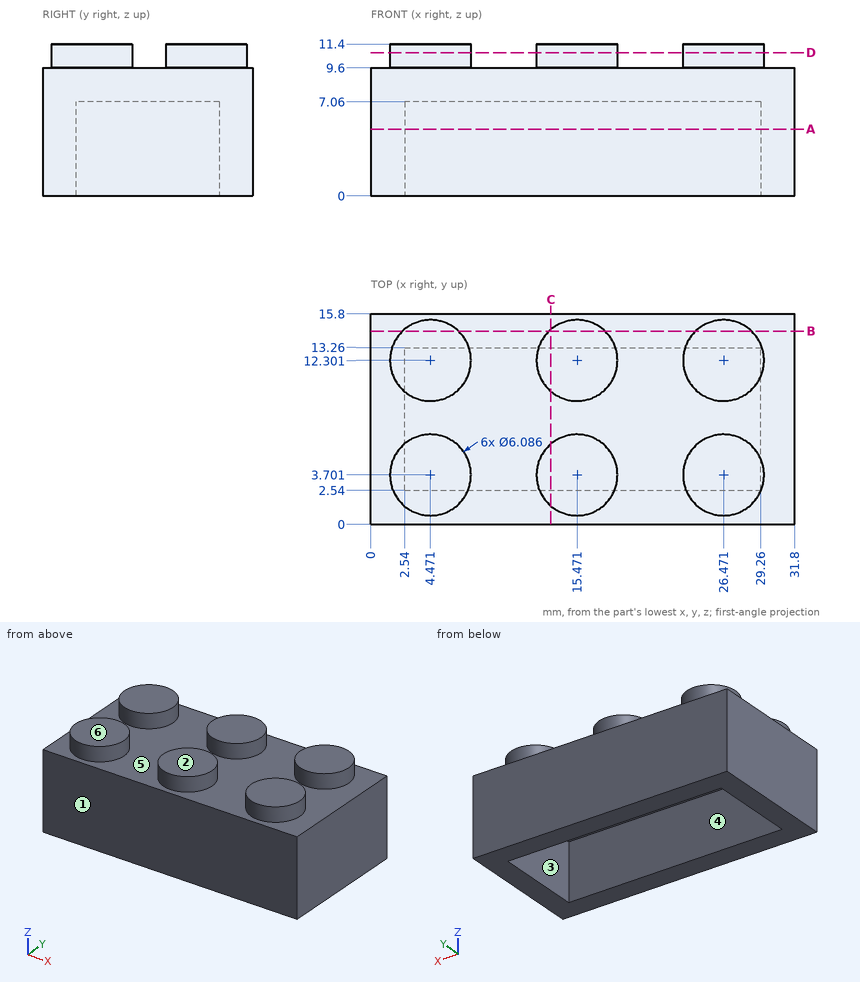
Can you work these out from the drawing? Everything is in mm from the part's minimum corner. A direction names the side the tool comes from. Round coordinates to 2 decimals unless told otherwise and drop trailing zeros. Loops run counter-clockwise (first coordinate to the right, second up) from the corner with the lowest first, then second, coordinate; pieces in that order, holes last. Notation, with made-up numbers: (14.5, 37.25) -> (44.5, 37.25) arc R29 cw to (44.5, 58.25) -> close; hole circle Ø6 at (-17, -39). An arc over 180 degrees is marked (long way). Answer in a Markdown table with one row per item.
Item 1: Will this pin go through, and if not, where does the flat tip stop? P1, Ø1, axis at x = 6.5, y = 7, coming from the -Z side.
Answer block:
| item | result |
|---|---|
| P1 | z = 7.06 |
Item 2: Suppose I cut it at D-D, the plane z = 10.75. List the corners of the cut face in (x, y) for me.
Answer block:
| item | result |
|---|---|
| outline | circle Ø6.09 at (4.47, 3.7); circle Ø6.09 at (4.47, 12.3); circle Ø6.09 at (15.47, 3.7); circle Ø6.09 at (15.47, 12.3); circle Ø6.09 at (26.47, 3.7); circle Ø6.09 at (26.47, 12.3) |
Item 3: If I drill on probe 1 along Y at (x, z) = (23.5, 5.75); probe 2 along X at (y, z) = (9, 6.5); probe 3 along X at (y, z) = (6, 10.5) (1 decimal), over which ranges is the centre line in solid material (lowest first)?
Answer block:
| item | result |
|---|---|
| probe 1 | 0 to 2.54, 13.26 to 15.8 |
| probe 2 | 0 to 2.54, 29.26 to 31.8 |
| probe 3 | 2.5 to 6.5, 13.5 to 17.5, 24.5 to 28.5 |
Item 4: Suppose I cut it at B-B, the plane y = 14.5. List the corners of the cut face in (x, z) for me (1 decimal), plus the area to 3 significant figures.
Answer block:
| item | result |
|---|---|
| outline | (0, 0) -> (31.8, 0) -> (31.8, 9.6) -> (28.6, 9.6) -> (28.6, 11.4) -> (24.4, 11.4) -> (24.4, 9.6) -> (17.6, 9.6) -> (17.6, 11.4) -> (13.4, 11.4) -> (13.4, 9.6) -> (6.6, 9.6) -> (6.6, 11.4) -> (2.4, 11.4) -> (2.4, 9.6) -> (0, 9.6) -> close |
| area | 328 mm² |
Item 5: Suppose I cut it at A-A, the plane z = 5. List the corners of the cut face in (x, y) for me, plus the area to 3 significant figures.
Answer block:
| item | result |
|---|---|
| outline | (0, 0) -> (31.8, 0) -> (31.8, 15.8) -> (0, 15.8) -> close; hole (2.54, 2.54) -> (29.26, 2.54) -> (29.26, 13.26) -> (2.54, 13.26) -> close |
| area | 216 mm² |
Item 6: Suppose I cut it at C-C, the plane x = 13.5. List the corners of the cut face in (y, z) for me.
Answer block:
| item | result |
|---|---|
| outline | (0, 0) -> (2.54, 0) -> (2.54, 7.06) -> (13.26, 7.06) -> (13.26, 0) -> (15.8, 0) -> (15.8, 9.6) -> (14.62, 9.6) -> (14.62, 11.4) -> (9.98, 11.4) -> (9.98, 9.6) -> (6.02, 9.6) -> (6.02, 11.4) -> (1.38, 11.4) -> (1.38, 9.6) -> (0, 9.6) -> close |
Item 7: We'd pull the mould along Y, two halves only. Please class the marked faces 1, 2 and 3: released by +Y, released by -Y, zero draft, split by the parting line, or undercut.
Answer block:
| item | result |
|---|---|
| face 1 | released by -Y |
| face 2 | zero draft |
| face 3 | undercut |
Item 8: On a 3-axis mill with a long thin cutter (end or side, diameter ignored), from which of +Z, -Z, +X, -X, +Y, -Y can I reach the whole of each face in a straight line? I mean the marked faces 4, 5 and 6. Say none if no direction works.
Answer block:
| item | result |
|---|---|
| face 4 | -Z |
| face 5 | +Z |
| face 6 | +Z, +X, -X, +Y, -Y |
